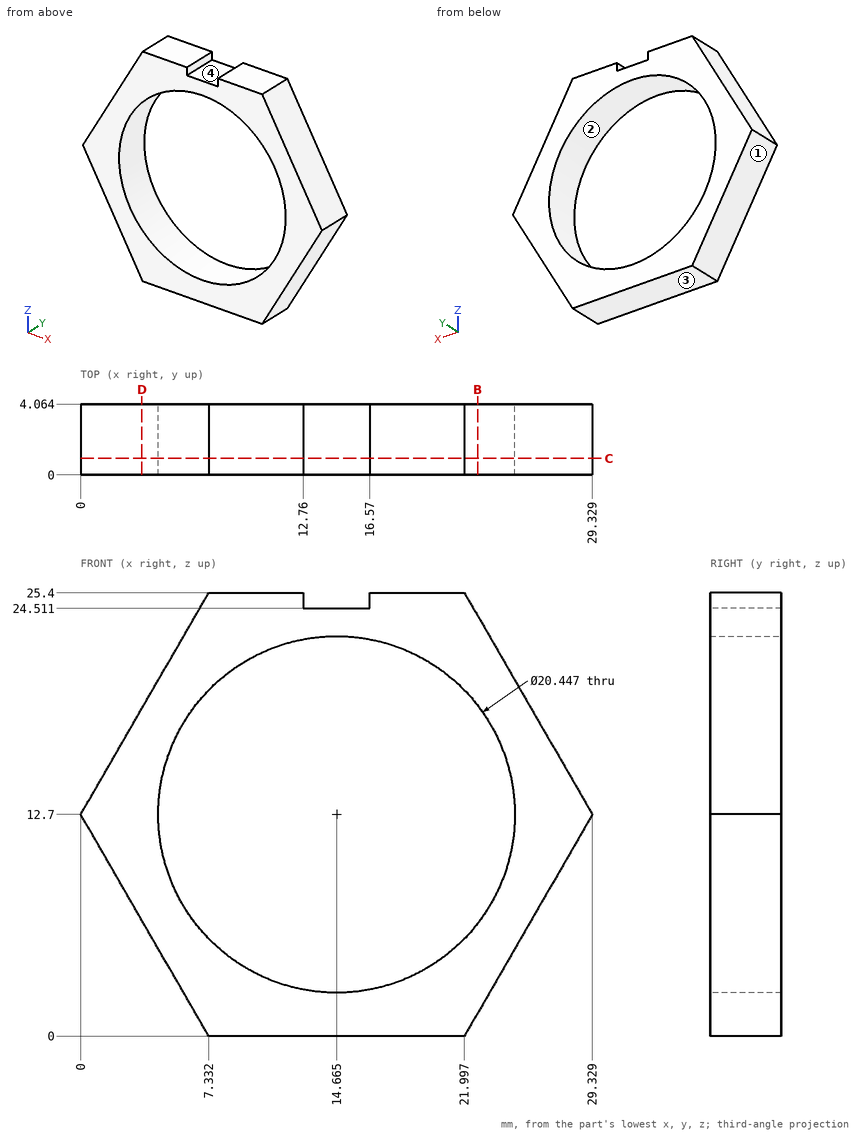
Can you work these out from the drawing? Everything is in mm from the part's minimum corner. Round coordinates to 2 decimals unless told otherwise and drop trailing zeros. Loops run counter-clockwise (first coordinate to the right, second up) from the corner with the lowest first, then second, coordinate; pieces in that order, holes last. Notation, with made-up numbers: (18, -29.5) -> (30, -29.5) arc R20 cw to (30, -8.5) -> close; hole circle Ø4 at (49.5, -17.75). An arc over 180 degrees is marked (long way). Put each result on its own line as item: value.
Q1. I want a section at B-B on x = 22.75. Write out the boundary of the cut face in (y, z).
Checks:
outline: (0, 1.3) -> (4.06, 1.3) -> (4.06, 6.44) -> (0, 6.44) -> close; (0, 18.96) -> (4.06, 18.96) -> (4.06, 24.1) -> (0, 24.1) -> close
Q2. Thinking about a two-plate mould opening in X: for the marked faces 1, 2, 3 and 4, which applies, pulls with the +X half, pulls with the -X half, needs draft (parallel to the pull), parting line crosses it, or undercut?
Checks:
face 1: pulls with the -X half
face 2: undercut
face 3: needs draft
face 4: undercut
Q3. Please list where these lines run through material, in increasing order: line 1 (Z direction, x = 22.5, y = 1.6) (1 decimal); line 2 (Z direction, x = 16, y = 3.6) (1 decimal); line 3 (X direction, y = 1.25, z = 13.5). Write a range as from..to.
Checks:
line 1: 0.9..6.1, 19.3..24.5
line 2: 0..2.6, 22.8..24.5
line 3: 0.46..4.47, 24.86..28.87
Q4. I want a section at C-C on y = 0.95. Write out the boundary of the cut face in (x, z) (1 decimal), and give its area (3 significant figures).
Checks:
outline: (0, 12.7) -> (7.3, 0) -> (22, 0) -> (29.3, 12.7) -> (22, 25.4) -> (16.6, 25.4) -> (16.6, 24.5) -> (12.8, 24.5) -> (12.8, 25.4) -> (7.3, 25.4) -> close; hole circle Ø20.4 at (14.7, 12.7)
area: 227 mm2
Q5. For pin 1 Ø1.5 at (y, z) = (2.5, 19.5) entering from +X; pin 2 Ø1.5 at (y, z) = (1.5, 11) entering from -X; pin 3 Ø1.9 at (x, y) = (15, 2.5) entering from +Z; pin 4 Ø1 at (x, z) = (13.5, 22) entering from +Y (1 decimal), each with a flat end and sliding along its axis, tell me the tip position at first contact or that it passes through.
Checks:
pin 1: x = 25.84
pin 2: x = 0.55
pin 3: z = 24.51
pin 4: through
Q6. I want a section at D-D on x = 3.5. Write out the boundary of the cut face in (y, z).
Checks:
outline: (0, 6.64) -> (4.06, 6.64) -> (4.06, 18.76) -> (0, 18.76) -> close
